Could you check a few things on this drawing? It's one solid part, dimensions in mm from its lowest x, y, z. Round coordinates to 2 decimals unless told otherwise and drop trailing zeros. Write each loop counter-clockwise with the first axis right and the second up, starting at its lowest first coordinate (ties: lowest second). Pieces come first, ordered by that corner, then holes. Notation, with made-up numbers: M -2,84.25 L 51,84.25 A29 ccw 51,107.25 Z; hole C 71.5,88.25 d4. An arc over 180 degrees is marked long. One line per item, written item: value. Start each with the question number.
(1) If I drill on L1, parallel to Y at x = 48, z = 3.55; L2, parallel to Y at x = 49, z = 0.75; L3, parallel to Z at x = 9.5, y = 47, over which ranges is the centre line in solid material (lowest first)?
(2) I want a section at A-A on y = 10. Please give me the cut outline in (x, z), and give its area (3 significant figures).
(3) I'm going to push flat-ended pins straight in: pin 1 Ø3.5 at (x, y) = (48, 49) entering from -Z; pin 2 Ø1.5 at (y, z) = (6, 1.5) entering from -X. Where does each tip first touch, or does it pass through?
(4) I want a section at C-C on z = 3.95. Please give me the cut outline in (x, y), and give its area (3 significant figures).
(5) I want a section at B-B on x = 48. Please give me the cut outline in (y, z), and give its area (3 significant figures).
(6) I want a section at D-D on y = 4. Please give me the cut outline in (x, z).
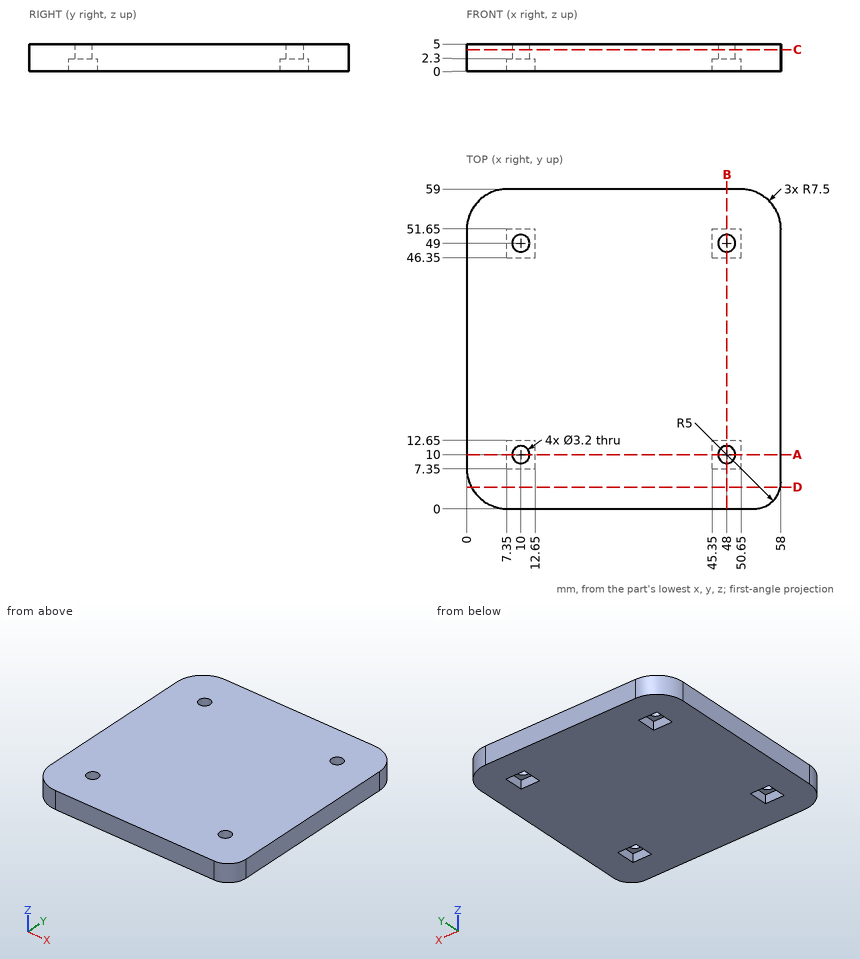
Found:
1. L1: y = 0 to 8.4, 11.6 to 47.4, 50.6 to 59
1. L2: y = 0 to 7.35, 12.65 to 46.35, 51.65 to 59
1. L3: z = 2.3 to 5
2. outline: M 0,0 L 7.35,0 L 7.35,2.3 L 8.4,2.3 L 8.4,5 L 0,5 Z; M 11.6,2.3 L 12.65,2.3 L 12.65,0 L 45.35,0 L 45.35,2.3 L 46.4,2.3 L 46.4,5 L 11.6,5 Z; M 49.6,2.3 L 50.65,2.3 L 50.65,0 L 58,0 L 58,5 L 49.6,5 Z
2. area: 248 mm²
3. pin 1: stops at z = 2.3
3. pin 2: stops at x = 0.04
4. outline: M 0,7.5 A7.5 ccw 7.5,0 L 53,0 A5 ccw 58,5 L 58,51.5 A7.5 ccw 50.5,59 L 7.5,59 A7.5 ccw 0,51.5 Z; hole C 10,10 d3.2; hole C 10,49 d3.2; hole C 48,10 d3.2; hole C 48,49 d3.2
4. area: 3,350 mm²
5. outline: M 0,0 L 7.35,0 L 7.35,2.3 L 8.4,2.3 L 8.4,5 L 0,5 Z; M 11.6,2.3 L 12.65,2.3 L 12.65,0 L 46.35,0 L 46.35,2.3 L 47.4,2.3 L 47.4,5 L 11.6,5 Z; M 50.6,2.3 L 51.65,2.3 L 51.65,0 L 59,0 L 59,5 L 50.6,5 Z
5. area: 253 mm²
6. outline: M 0.87,0 L 57.9,0 L 57.9,5 L 0.87,5 Z
